Build history of the part. All positions in model axes, mm. Give positions to 0.01 mm unless a question says otherwise; leave off trailing zeros. Loops run counter-clockwise (first coordinate to the right, second up) from the corner with the lowest first, then second, coordinate; pieces in that order, holes last. Notation, with made-up numbers: M 86,86.5 L 144,86.5 A21 ccw 144,114.5 Z; hole C 14.25,70 d2. An arc over 180 degrees is marked long. Answer as a JSON object with one key per item and string values. Group by question number.
1. Drill centre lines: line 1 along Z through (x, y) = (107.95, -1); line 2 along X through (y, z) = (-1.1, -62); line 3 along Z through (x, y) = (10.16, -1.2). Where is each one in solid material? Low to high. Write a range as [from, to].
2. Slice it at C-C (y = -0.9). Give the number of separate pieces and of enclosed holes in the cut face, then the cut area to 3 significant figures.
3. Slice it at D-D (x = 205.74). List the corners of the cut face in (y, z), then the cut area to 3 significant figures.
4. Slice it at A-A (x = 107.95). List the corners of the cut face in (y, z).
5. Slice it at B-B (z = -57.15). List the corners of the cut face in (x, y), then the cut area to 3 significant figures.
6. Drop flat-ended pins along their axis: pin 1 Ø5 at (x, z) = (33.21, -66.65) entering from -Y; pin 2 Ø19 at (x, z) = (45.212, -57.15) entering from -Y. Give the stop position or say it passes through.
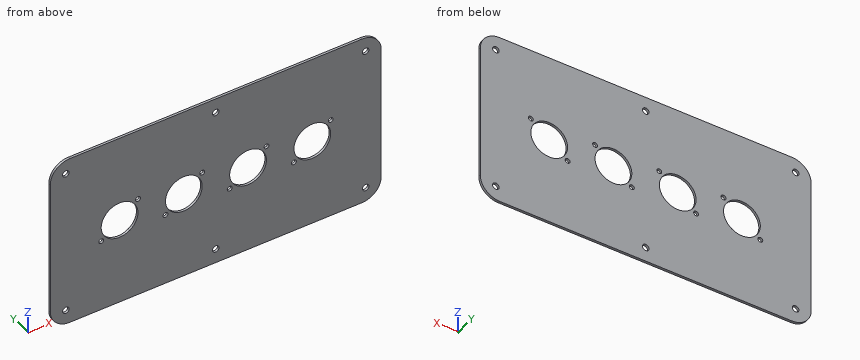
from build123d import *

# Parameters (mm, degrees)
F1_DEPTH = 1.524
F2_R     = 12.0015
F2_R_2   = 1.6002
F3_DEPTH = 1.525
F5_D     = 4.318


with BuildPart() as f1:
    # F0 (on Front) → F1 (new body)
    with BuildSketch(Plane.XZ):
        with BuildLine():
            Line((203.2, 0), (12.7, 0))
            ThreePointArc((12.7, 0), (3.7197438789, -3.7197438789), (0, -12.7))
            Line((0, -12.7), (0, -101.6))
            ThreePointArc((0, -101.6), (3.7197438789, -110.5802561211), (12.7, -114.3))
            Line((12.7, -114.3), (203.2, -114.3))
            ThreePointArc((203.2, -114.3), (212.1802561211, -110.5802561211), (215.9, -101.6))
            Line((215.9, -101.6), (215.9, -12.7))
            ThreePointArc((215.9, -12.7), (212.1802561211, -3.7197438789), (203.2, 0))
        make_face()
    extrude(amount=F1_DEPTH)

    # F2 (on face) → F3 (cut, through all)
    with BuildSketch(Plane.XZ.offset(1.524)):
        with Locations((45.212, -57.15)):
            Circle(F2_R)
        with Locations((33.2105027356, -66.6496)):
            Circle(F2_R_2)
        with Locations((57.2135027356, -47.6504)):
            Circle(F2_R_2)
        with Locations((99.1235027356, -47.6504)):
            Circle(F2_R_2)
        with Locations((87.122, -57.15)):
            Circle(F2_R)
        with Locations((75.1205027356, -66.6496)):
            Circle(F2_R_2)
        with Locations((141.0335027356, -47.6504)):
            Circle(F2_R_2)
        with Locations((129.032, -57.15)):
            Circle(F2_R)
        with Locations((117.0305027356, -66.6496)):
            Circle(F2_R_2)
        with Locations((182.9435027356, -47.6504)):
            Circle(F2_R_2)
        with Locations((170.942, -57.15)):
            Circle(F2_R)
        with Locations((158.9405027356, -66.6496)):
            Circle(F2_R_2)
    extrude(amount=-F3_DEPTH, mode=Mode.SUBTRACT)

    # F5 (through all)
    with Locations(Plane.XZ.offset(1.524)):
        with Locations((10.16, -9.525), (107.95, -9.525), (205.74, -9.525), (205.74, -104.775), (107.95, -104.775), (10.16, -104.775)):
            Hole(F5_D / 2)


solid = f1.part
Established:
{
 "1": {"line 1": "z = [-114.3, -106.93], [-102.62, -11.68], [-7.37, 0]", "line 2": "x = [0, 34.23], [56.19, 76.14], [98.1, 118.05], [140.01, 159.96], [181.92, 215.9]", "line 3": "z = [-114.04, -106.93], [-102.62, -11.68], [-7.37, -0.26]"},
 "2": {"separate pieces": "1", "enclosed holes": "18", "area": "22,600 mm^2"},
 "3": {"outline": "M -1.52,-114.04 L 0,-114.04 L 0,-106.93 L -1.52,-106.93 Z; M -1.52,-102.62 L 0,-102.62 L 0,-11.68 L -1.52,-11.68 Z; M -1.52,-7.37 L 0,-7.37 L 0,-0.26 L -1.52,-0.26 Z", "area": "160 mm^2"},
 "4": {"outline": "M -1.52,-114.3 L 0,-114.3 L 0,-106.93 L -1.52,-106.93 Z; M -1.52,-102.62 L 0,-102.62 L 0,-11.68 L -1.52,-11.68 Z; M -1.52,-7.37 L 0,-7.37 L 0,0 L -1.52,0 Z"},
 "5": {"outline": "M 0,-1.52 L 33.21,-1.52 L 33.21,0 L 0,0 Z; M 57.21,-1.52 L 75.12,-1.52 L 75.12,0 L 57.21,0 Z; M 99.12,-1.52 L 117.03,-1.52 L 117.03,0 L 99.12,0 Z; M 141.03,-1.52 L 158.94,-1.52 L 158.94,0 L 141.03,0 Z; M 182.94,-1.52 L 215.9,-1.52 L 215.9,0 L 182.94,0 Z", "area": "183 mm^2"},
 "6": {"pin 1": "stops at y = -1.52", "pin 2": "passes through"}
}
